The figure shows three views and two pictorial views of one solid part (mm, origin at its lowest corner). Answer the questions. A direction names the side the tool comes from. Give positions to 0.01 mm unless a question says otherwise; leave off trailing zeros. Loops run counter-clockwise (first coordinate to the right, second up) from the corner with the lowest first, then second, coordinate; pieces in that order, holes last. Notation, with made-up numbers: M -14.5,-26.5 L 8.5,-26.5 A32 ccw 8.5,2.5 Z; hole C -38.75,-1.75 d5. An arc over 180 degrees is marked long. Write item = value, one per line. Start each with the question number.
1. Section A-A on y = 13 is taken. Determine the outline of the cut face in (x, z) (3 decimals), plus the area to 3 significant figures.
2. Section D-D on z = 1 is taken. Determine the outline of the cut face in (x, y) (3 decimals), plus the area to 3 significant figures.
3. Section C-C on z = 4 is taken. Determine the outline of the cut face in (x, y) (3 decimals).
4. Consider L1, parallel to Y at x = 13, z = 3.25 (3 decimals); L2, parallel to Y at x = 13, z = 5.25 (3 decimals); L3, parallel to Z at x = 2.25, y = 10.5. Determine where each line is inside the solid, lowest interval first. Write a range as [from, to].
5. The mould has two halves that part along X. Classify the marked faces 1, 2 and 3: released by +X, released by -X, zero draft, split by the parting line, or undercut.
6. Flat-ended cylindrical pins translate along their axes: pin 1 Ø1.5 at (x, y) = (15.5, 23) entering from +Z; pin 2 Ø2 at (x, y) = (13, 13) entering from -Z (3 decimals); pin 3 Ø3 at (x, z) = (21.5, 1) entering from +Y; pin 4 Ø1 at (x, z) = (19.5, 4.5) entering from -Y. Find the tip coordinate at first contact, or state that the pin passes through.
7. For the marked faces 4 and 5, determine the directions among +Z, -Z, +X, -X, +Y, -Y from which every point of the face is accessible in a straight line to the end or side of a thin tool.
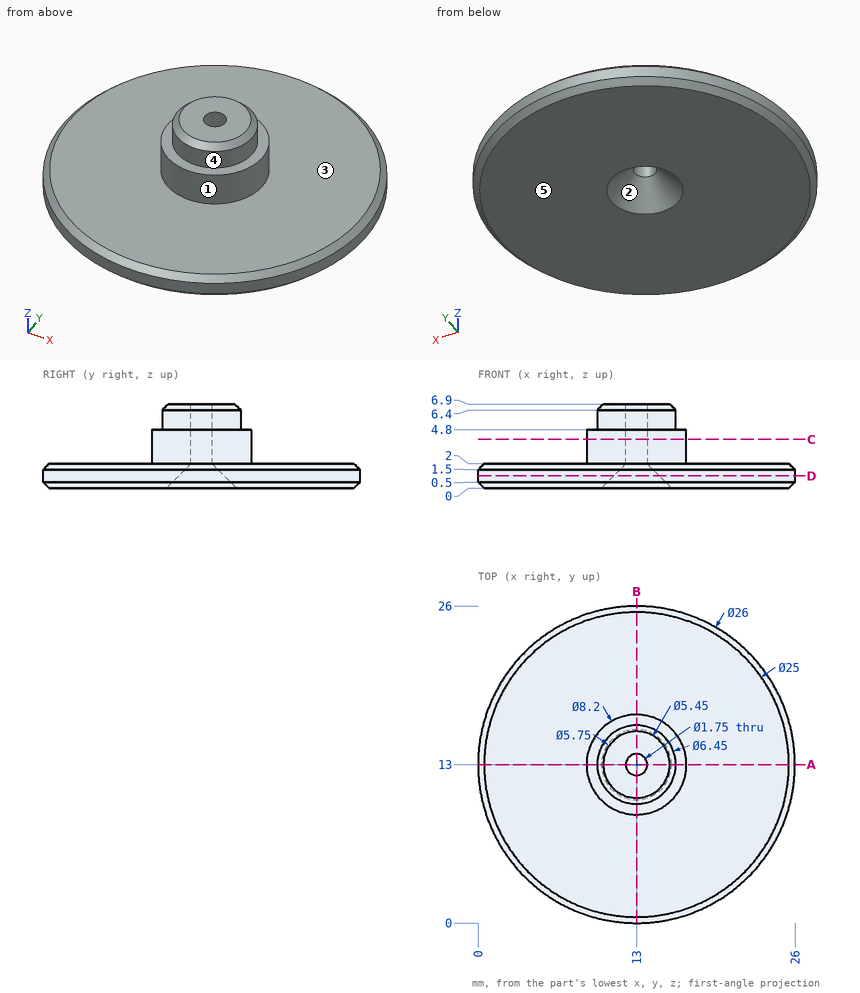
Verdict:
q1.outline = M 0,0.5 L 0.5,0 L 10.125,0 L 12.125,2 L 12.125,6.9 L 10.275,6.9 L 9.775,6.4 L 9.775,4.8 L 8.9,4.8 L 8.9,2 L 0.5,2 L 0,1.5 Z; M 13.875,2 L 15.875,0 L 25.5,0 L 26,0.5 L 26,1.5 L 25.5,2 L 17.1,2 L 17.1,4.8 L 16.225,4.8 L 16.225,6.4 L 15.725,6.9 L 13.875,6.9 Z
q1.area = 71.7 mm2
q2.outline = C 13,13 d26; hole C 13,13 d3.75
q2.area = 520 mm2
q3.outline = C 13,13 d8.2; hole C 13,13 d1.75
q4.L1 = [8.9, 12.125], [13.875, 17.1]
q4.L2 = [9.775, 12.125], [13.875, 16.225]
q4.L3 = [0, 2]
q5.face_1 = split by the parting line
q5.face_2 = undercut
q5.face_3 = zero draft
q6.pin_1 = 2
q6.pin_2 = 1.875
q6.pin_3 = 23.95
q6.pin_4 = through
q7.face_4 = +Z
q7.face_5 = -Z, +X, -X, +Y, -Y
